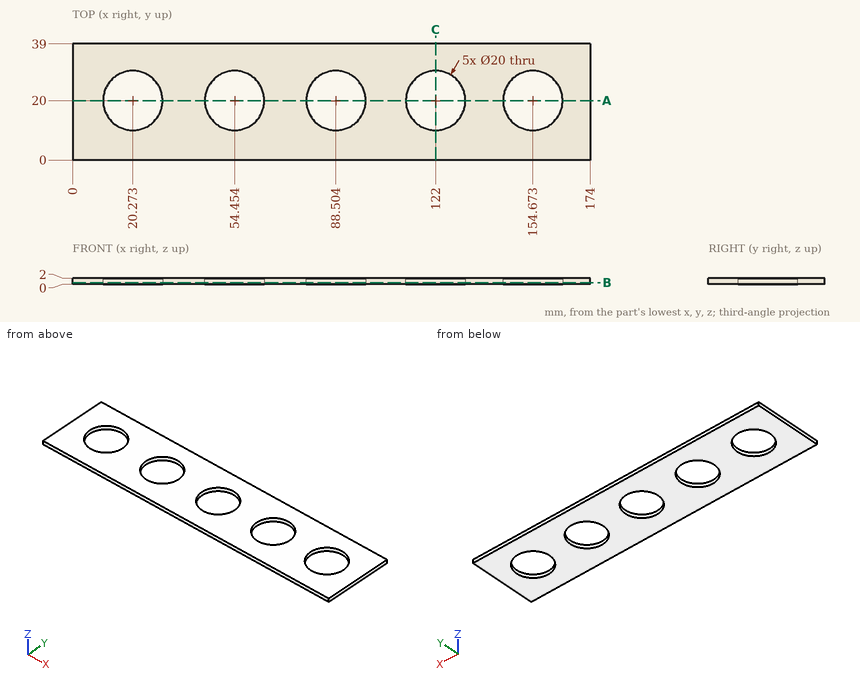
Geometry: see drawing. Coordinates: mm, zero at the bounding-box minimum. Give positions to 0.01 mm unless a question says otherwise; leave off trailing zeros. Loops run counter-clockwise (first coordinate to the right, second up) from the corner with the lowest first, then second, coordinate; pieces in that order, holes last. Notation, with made-up numbers: (-8.75, 43) -> (17.25, 43) arc R16 cw to (17.25, 62) -> close; hole circle Ø4 at (62, -8). An arc over 180 degrees is marked (long way). Answer as a JSON object with one key per item and string values. Group by question number.
Item 1: Line query: probe 1 along X at (y, z) = (12, 0.75) (1 decimal); probe 2 along X at (y, z) = (12.5, 0.5) (1 decimal); probe 3 along Y at (x, z) = (149, 0.55) (1 decimal). Output: solid intervals per line, ascending.
Item 2: Cut plane A-A, the plane y = 20. Return the cut outline in (x, z) (1 decimal), and give its area (3 significant figures).
Item 3: Cut plane C-C, the plane x = 122. Return the cut outline in (y, z).
Item 4: Cut plane B-B, the plane z = 0.45. Return the cut outline in (x, y) (1 decimal).
Checks:
{
 "1": {"probe 1": "x = 0 to 14.3, 26.3 to 48.5, 60.5 to 82.5, 94.5 to 116, 128 to 148.7, 160.7 to 174", "probe 2": "x = 0 to 13.7, 26.9 to 47.8, 61.1 to 81.9, 95.1 to 115.4, 128.6 to 148.1, 161.3 to 174", "probe 3": "y = 0 to 11.8, 28.2 to 39"},
 "2": {"outline": "(0, 0) -> (10.3, 0) -> (10.3, 2) -> (0, 2) -> close; (30.3, 0) -> (44.5, 0) -> (44.5, 2) -> (30.3, 2) -> close; (64.5, 0) -> (78.5, 0) -> (78.5, 2) -> (64.5, 2) -> close; (98.5, 0) -> (112, 0) -> (112, 2) -> (98.5, 2) -> close; (132, 0) -> (144.7, 0) -> (144.7, 2) -> (132, 2) -> close; (164.7, 0) -> (174, 0) -> (174, 2) -> (164.7, 2) -> close", "area": "148 mm²"},
 "3": {"outline": "(0, 0) -> (10, 0) -> (10, 2) -> (0, 2) -> close; (30, 0) -> (39, 0) -> (39, 2) -> (30, 2) -> close"},
 "4": {"outline": "(0, 0) -> (174, 0) -> (174, 39) -> (0, 39) -> close; hole circle Ø20 at (20.3, 20); hole circle Ø20 at (54.5, 20); hole circle Ø20 at (88.5, 20); hole circle Ø20 at (122, 20); hole circle Ø20 at (154.7, 20)"}
}
